```python
from build123d import *

# Parameters (mm, degrees)
SKETCH2_R           = 2.5527
SKETCH2_R_2         = 11.176
BOSS_EXTRUDE1_DEPTH = 3.175


with BuildPart() as part:
    # Sketch2 → Boss-Extrude1 (new body)
    with BuildSketch(Plane.XY):
        with BuildLine():
            Line((89.804840449, 162.158224077), (133.35, 162.158224077))
            ThreePointArc((133.35, 162.158224077), (137.840128061, 160.298352138), (139.7, 155.808224077))
            Line((139.7, 155.808224077), (139.7, 93.800599977))
            ThreePointArc((139.7, 93.800599977), (138.794482451, 88.24423856), (136.171639749, 83.262892317))
            Line((136.171639749, 83.262892317), (125.655155155, 69.319391612))
            ThreePointArc((125.655155155, 69.319391612), (122.975635879, 67.362639494), (119.660773298, 67.219851313))
            Line((119.660773298, 67.219851313), (96.672878026, 73.109258508))
            ThreePointArc((96.672878026, 73.109258508), (89.283742308, 78.328372298), (87.243120334, 87.141676865))
            ThreePointArc((87.243120334, 87.141676865), (88.644839635, 120.88029943), (83.642604572, 154.275465457))
            ThreePointArc((83.642604572, 154.275465457), (84.802065357, 159.719073266), (89.804840449, 162.158224077))
        make_face()
        with Locations((89.657841737, 156.395094021)):
            Circle(SKETCH2_R, mode=Mode.SUBTRACT)
        with Locations((91.747700228, 147.102187237)):
            Circle(SKETCH2_R, mode=Mode.SUBTRACT)
        with Locations((106.775437357, 76.433708644)):
            Circle(SKETCH2_R, mode=Mode.SUBTRACT)
        with Locations((115.1001, 121.545060726)):
            Circle(SKETCH2_R_2, mode=Mode.SUBTRACT)
        with Locations((113.962375762, 145.648224077)):
            Circle(SKETCH2_R_2, mode=Mode.SUBTRACT)
        with Locations((133.35, 155.808224077)):
            Circle(SKETCH2_R, mode=Mode.SUBTRACT)
        with Locations((121.082277384, 72.768353221)):
            Circle(SKETCH2_R, mode=Mode.SUBTRACT)
        with Locations((121.082277384, 98.168353221)):
            Circle(SKETCH2_R_2, mode=Mode.SUBTRACT)
    extrude(amount=BOSS_EXTRUDE1_DEPTH)


solid = part.part
```
Read the model definition and answer for the solid it produces. Units are mm, in the model's axes. Give positions to 0.01 mm unless a question says otherwise; leave off trailing zeros. Write each loop counter-clockwise with the first axis right and the second up, starting at its lowest first coordinate (ties: lowest second). Pieces come first, ordered by that corner, then holes. Notation, with made-up numbers: (22.5, 70) -> (69.5, 70) arc R15 ccw to (69.5, 95) -> close; hole circle Ø1 at (28.5, -12). An arc over 180 degrees is marked (long way). Answer in a Markdown table with one row per item.
1) Section A-A on y = 95 is taken. Give the vertices of the cut face in (x, z) (3 decimals), plus the area to 3 significant figures.
Results list:
| item | result |
|---|---|
| outline | (88.146, 0) -> (110.365, 0) -> (110.365, 3.175) -> (88.146, 3.175) -> close; (131.8, 0) -> (139.7, 0) -> (139.7, 3.175) -> (131.8, 3.175) -> close |
| area | 95.6 mm^2 |
2) Straight lines are drawn through the part: line 1 (Y direction, x = 111, z = 1.7); line 2 (Y direction, x = 91, z = 2.1); line 3 (Y direction, x = 106, z = 2.7). For each, find the intervals that lie inside material, in ascending order. Write a range as [from, to].
Results list:
| item | result |
|---|---|
| line 1 | [69.44, 93.35], [102.99, 111.15], [131.94, 134.87], [156.42, 162.16] |
| line 2 | [76.28, 144.66], [149.54, 154.22], [158.57, 162.16] |
| line 3 | [70.72, 74], [78.87, 115.06], [128.03, 137.81], [153.49, 162.16] |
3) Section B-B on x = 113 is taken. Give the vertices of the cut face in (y, z) (3 decimals), plus the area to 3 significant figures.
Results list:
| item | result |
|---|---|
| outline | (68.926, 0) -> (90.45, 0) -> (90.45, 3.175) -> (68.926, 3.175) -> close; (105.887, 0) -> (110.568, 0) -> (110.568, 3.175) -> (105.887, 3.175) -> close; (132.522, 0) -> (134.514, 0) -> (134.514, 3.175) -> (132.522, 3.175) -> close; (156.783, 0) -> (162.158, 0) -> (162.158, 3.175) -> (156.783, 3.175) -> close |
| area | 107 mm^2 |
4) Determine the mould class of faces 1 (the cylindrical face through (138.82, 88.32, 1.57)), 2 (the cylindrical face through (93.12, 149.255, 1.565)), 3 (the flat face through (139.7, 125, 2)) for opening direction Y: released by +Y, released by -Y, zero draft, split by the parting line, or undercut.
Results list:
| item | result |
|---|---|
| face 1 | released by -Y |
| face 2 | undercut |
| face 3 | zero draft |
5) Each of these flat-tipped pins is pushed along its axis until it touches: pin 1 Ø18 at (x, y) = (113.96, 145.65) entering from -Z; pin 2 Ø1.5 at (y, z) = (135.5, 2) entering from -X. Where does it stop, or does it pass through?
Results list:
| item | result |
|---|---|
| pin 1 | through |
| pin 2 | x = 87.15 |
6) Section C-C on z = 1.6 is taken. Count the separate pieces of the cut face and the enclosed holes in it, plus the area to 3 significant figures.
Results list:
| item | result |
|---|---|
| separate pieces | 1 |
| enclosed holes | 8 |
| area | 3,370 mm^2 |
7) Section D-D on y = 105.5 is taken. Give the vertices of the cut face in (x, z) (3 decimals).
Results list:
| item | result |
|---|---|
| outline | (88.803, 0) -> (112.647, 0) -> (112.647, 3.175) -> (88.803, 3.175) -> close; (129.517, 0) -> (139.7, 0) -> (139.7, 3.175) -> (129.517, 3.175) -> close |
